Could you check a few things on this drawing? It's one solid part, dimensions in mm from its lowest x, y, z. A direction names the side the tool comes from. Round coordinates to 2 decimals unless told otherwise and drop trailing zeros. Write each loop counter-clockwise with the first axis right and the second up, starting at its lowest first coordinate (ties: lowest second). Pieces come first, ordered by that corner, then holes. Notation, with made-up numbers: (15, 13) -> (64, 13) arc R32 cw to (64, 50) -> close; hole circle Ø2 at (-39.5, 15). An arc over 180 degrees is marked (long way). Put each result on its own line as item: value. Start each with the question number.
1) Will this pin go through, and if not, where does the flat tip stop? P1, Ø3.5, axis at x = 4, z = 24.5, coming from the -Y side.
2) I want a section at C-C, the plane z = 2.5. List the corners of the cut face in (x, y) for me, then the cut area to 3 significant figures.
3) Which directions (+Z, -Z, +X, -X, +Y, -Y) give clear straight access to the entire face, cutting with the end or side of a thin tool? Please do the marked faces 1 and 2.
4) I want a section at D-D, the plane x = 8.5. List the corners of the cut face in (y, z) for me (1 decimal), then the cut area to 3 significant figures.
5) I want a section at B-B, the plane y = 11. List the corners of the cut face in (x, z) for me.
6) If I drill on line 1 along X through (y, z) = (6, 12.5); line 2 along Y through (x, z) = (4.5, 11.75) (1 decimal); line 3 along Y through (x, z) = (3.5, 8.5) (1 decimal), over which ranges is the centre line in solid material (lowest first)? Write a range as [from, to].
7) I want a section at A-A, the plane x = 9.75. List the corners of the cut face in (y, z) for me (1 decimal).
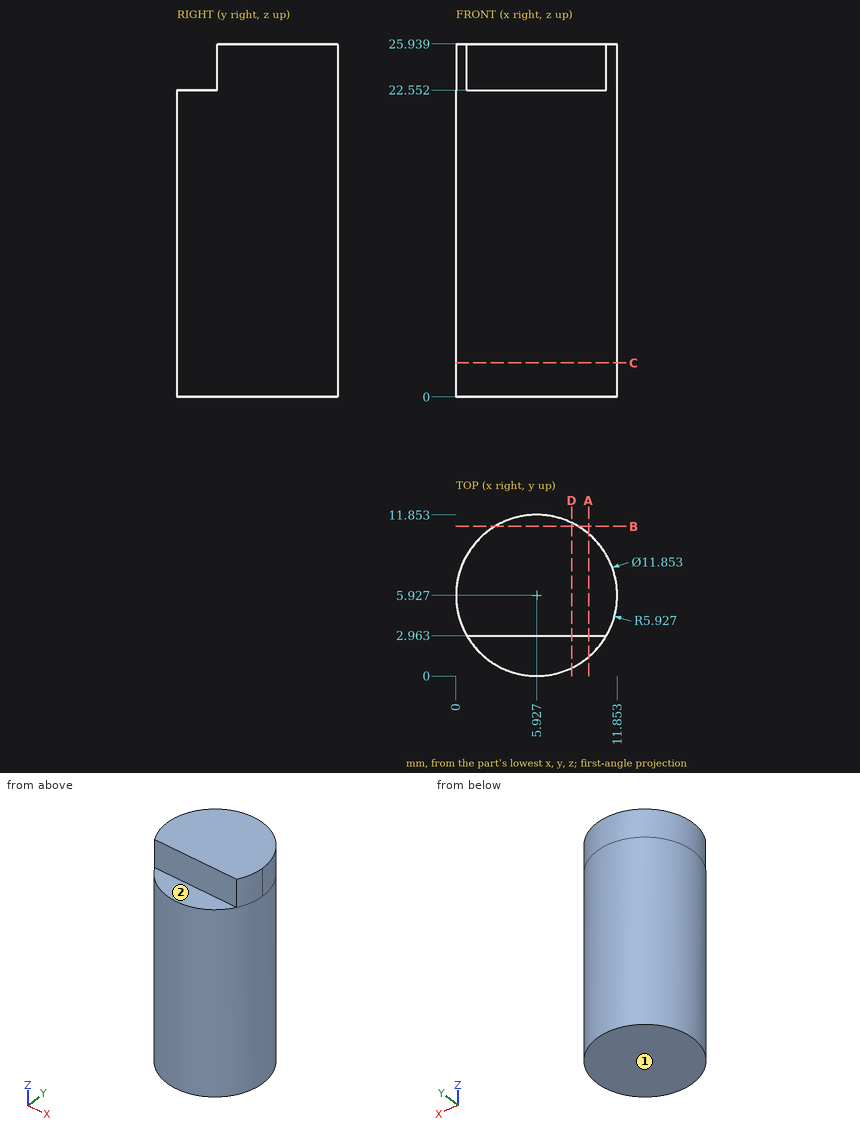
Findings:
1. P1: stops at y = 2.96
2. outline: circle Ø11.85 at (5.93, 5.93)
2. area: 110 mm2
3. face 1: -Z, +X, -X, +Y, -Y
3. face 2: +Z, +X, -X, -Y
4. outline: (0.6, 0) -> (11.3, 0) -> (11.3, 25.9) -> (3, 25.9) -> (3, 22.6) -> (0.6, 22.6) -> close
4. area: 269 mm2
5. outline: (2.86, 0) -> (8.99, 0) -> (8.99, 25.94) -> (2.86, 25.94) -> close
6. line 1: x = [0, 11.85]
6. line 2: y = [0.2, 11.7]
6. line 3: y = [0.5, 11.3]
7. outline: (1.4, 0) -> (10.5, 0) -> (10.5, 25.9) -> (3, 25.9) -> (3, 22.6) -> (1.4, 22.6) -> close
